Build history of the part. All positions in model axes, mm. Round coordinates to 2 decimals unless told otherwise and drop trailing zeros. Write each loop counter-clockwise with the first axis right and the second up, starting at its lowest first coordinate (ties: lowest second). Pieces come first, ordered by that corner, then holes. Notation, with made-up numbers: M 16,-14 L 42,-14 A7 ccw 42,-1 Z; hole C 73,6.25 d9. An arc over 180 degrees is marked long. Write item = value, one per line.
from build123d import *

# Parameters (mm, degrees)
F0_R      = 1.5
F1_DEPTH  = 15
F0_R_2    = 17.5
F2_SIZE   = 1.5
F2_2_SIZE = 1.5


with BuildPart() as f1:
    # F0 (on Top) → F1 (new body)
    with BuildSketch(Plane.XY):
        with Locations((-49.0162223577, 3.6474848166)):
            Circle(F0_R)
    extrude(amount=F1_DEPTH)

    # F2
    f2_edges = [f1.edges().sort_by_distance(p)[0] for p in [
        (-50.516222, 3.647485, 15),
    ]]
    chamfer(f2_edges, length=F2_SIZE)


with BuildPart() as f1b:
    # F0 (on Top) → F1, piece 2 (new body)
    with BuildSketch(Plane.XY):
        Circle(F0_R_2)
    extrude(amount=F1_DEPTH)

    # F2#2
    f2_2_edges = [f1b.edges().sort_by_distance(p)[0] for p in [
        (-17.5, 0, 15),
        (17.5, 0, 7.5),
        (-17.5, 0, 0),
    ]]
    chamfer(f2_2_edges, length=F2_2_SIZE)


solid = f1b.part
1. Band-saw the part on A-A (z = 4). List the corners of the cut face in (x, y), plus the area to 3 significant figures.
Responses:
outline = C 0,0 d35
area = 962 mm²
2. Flat gauge pins, fed straight in: pin 1 (5 mm diameter, centred on y = -9, z = 10, fed in from -X); pin 2 (2 mm diameter, centred on x = 10, z = 13.5, fed in from +Y); pin 3 (1 mm diameter, centred on y = 2, z = 6.5, fed in from -X). Where does each tip first touch, or does it go through?
Responses:
pin_1 = -16.25
pin_2 = 15.01
pin_3 = -17.44
3. Probe probe 1 along Y at (x, z) = (-11, 3.5); probe 2 along Y at (x, z) = (-15, 11.5); probe 3 along X at (y, z) = (7, 6.5). List the from-to ranges inside material, lowest first.
Responses:
probe_1 = -13.61 to 13.61
probe_2 = -9.01 to 9.01
probe_3 = -16.04 to 16.04
